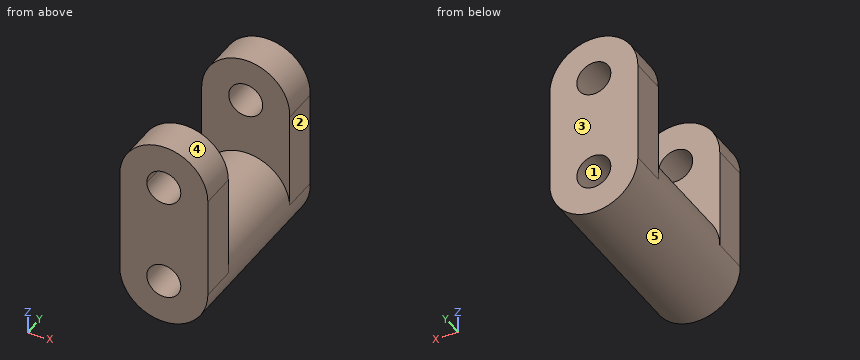
from build123d import *

# Parameters (mm, degrees)
F0_R     = 29.837596
F1_DEPTH = 127
F3_DEPTH = 25.4
F5_DEPTH = 25.4
F6_R     = 11.514098
F7_DEPTH = 249.174


with BuildPart() as f1:
    # F0 (on Front) → F1 (new body)
    with BuildSketch(Plane.XZ):
        with Locations((0, -34.119722)):
            Circle(F0_R)
    extrude(amount=F1_DEPTH)

    # F2 (on face) → F3 (join)
    with BuildSketch(Plane.XZ.offset(127)):
        with BuildLine():
            Line((-11.514098, -34.119722), (0, -34.119722))
            Line((0, -34.119722), (11.514098, -34.119722))
            ThreePointArc((11.514098, -34.119722), (0, -22.605623), (-11.514098, -34.119722))
        make_face()
        with BuildLine():
            Line((-29.837596, -34.119722), (-11.514098, -34.119722))
            ThreePointArc((-11.514098, -34.119722), (0, -22.605623), (11.514098, -34.119722))
            Line((11.514098, -34.119722), (29.837596, -34.119722))
            ThreePointArc((29.837596, -34.119722), (0, -4.282125), (-29.837596, -34.119722))
        make_face()
        with BuildLine():
            Line((-29.837596, 34.119722), (-29.837596, -34.119722))
            ThreePointArc((-29.837596, -34.119722), (0, -4.282125), (29.837596, -34.119722))
            Line((29.837596, -34.119722), (29.837596, 34.119722))
            ThreePointArc((29.837596, 34.119722), (0, 63.957318), (-29.837596, 34.119722))
        make_face()
        with BuildLine():
            ThreePointArc((11.514098, 34.119722), (0, 22.605623), (-11.514098, 34.119722))
            ThreePointArc((-11.514098, 34.119722), (0, 45.63382), (11.514098, 34.119722))
        make_face(mode=Mode.SUBTRACT)
    extrude(amount=-F3_DEPTH)

    # F4 (on face) → F5 (join)
    with BuildSketch(Plane(origin=(0, 0, 0), x_dir=(-1, 0, 0), z_dir=(0, 1, 0))):
        with BuildLine():
            Line((-29.798884, -34.119722), (0, -34.119722))
            Line((0, -34.119722), (29.416961, -34.119722))
            Line((29.416961, -34.119722), (29.837596, -34.119722))
            Line((29.837596, -34.119722), (29.837596, -29.127271))
            Line((29.837596, -29.127271), (29.837596, 33.523746))
            ThreePointArc((29.837596, 33.523746), (-0.759963, 63.351663), (-29.798884, 32.004312))
            Line((-29.798884, 32.004312), (-29.798884, -34.119722))
        make_face()
    extrude(amount=-F5_DEPTH)

    # F6 (on face) → F7 (cut)
    with BuildSketch(Plane.XZ.offset(127)):
        with Locations((0, 34.119722)):
            Circle(F6_R)
        with Locations((0, -34.119722)):
            Circle(F6_R)
    extrude(amount=-F7_DEPTH, mode=Mode.SUBTRACT)


solid = f1.part
Check sheet for the modelled part. Datum: model origin and axes. Units: mm. Face numbers are marked on the shaded views. A direction names the side the tool comes from. Give positions to 0.01 mm unless a question says otherwise; leave off trailing zeros. Write each loop counter-clockwise with the first axis right and the second up, starting at its lowest first coordinate (ties: lowest second). Pieces come first, ordered by that corner, then holes. Notation, with made-up numbers: (84.25, 9) -> (114.25, 9) arc R16 ccw to (114.25, 18) -> close; hole circle Ø3 at (67.5, 17). An arc over 180 degrees is marked (long way). Use one line per item in the form item = value. Start each with the question number.
1. Go/stop test with flat-tipped pins: P1, Ø10, axis at x = 11.5, y = -104, coming from the +Z side; P2, Ø3, axis at x = 20.5, y = -69, coming from the -Z side; P3, Ø20.5, axis at x = 0, z = 34.12, coming from the +Y side; P4, Ø6, axis at x = -4.5, y = -21.5, coming from the +Z side. Record where each tip stops, or that it passes through.
2. Section check A-A (x = 0). Record the cut outline in (y, z), and give its area (3 significant figures).
3. Section check B-B (z = 14.5). Record the cut outline in (x, y).
4. Section check D-D (z = 55). Record the cut outline in (x, y).
5. Section check C-C (y = -20.5). Record the cut outline in (x, z).
6. Thickness scan on line 1 along Z through (x, y) = (0, -74); line 2 along Y through (x, z) = (-13.5, 57.5); line 3 along Z through (x, y) = (0, -18.5). Record the ranges inside material, lowest first. Write a range as from..to.
7. Mould release check, pull along X, two halves, no side actions. Record for the marked faces 1, 2 and 3: pulls with the +X half, pulls with the -X half, needs draft (parallel to the pull), parting line crosses it, or undercut.
8. Access from +Z, -Z, +X, -X, +Y, -Y to the whole of each face (thin tool, end or side, straight path). Record for the marked faces 4 and 5.
Conclusion:
q1.P1 = 63.24
q1.P2 = -57.13
q1.P3 = through
q1.P4 = 63.32
q2.outline = (-127, -63.96) -> (0, -63.96) -> (0, -45.63) -> (-127, -45.63) -> close; (-127, -22.61) -> (0, -22.61) -> (0, 22.61) -> (-25.4, 22.61) -> (-25.4, -4.28) -> (-101.6, -4.28) -> (-101.6, 22.61) -> (-127, 22.61) -> close; (-127, 45.63) -> (-101.6, 45.63) -> (-101.6, 63.96) -> (-127, 63.96) -> close; (-25.4, 45.63) -> (0, 45.63) -> (0, 63.36) -> (-25.4, 63.36) -> close
q2.area = 6,940 mm²
q3.outline = (-29.84, -127) -> (29.84, -127) -> (29.84, -101.6) -> (-29.84, -101.6) -> close; (-29.84, -25.4) -> (29.8, -25.4) -> (29.8, 0) -> (-29.84, 0) -> close
q4.outline = (-21.31, -127) -> (21.31, -127) -> (21.31, -101.6) -> (-21.31, -101.6) -> close; (-20.71, -25.4) -> (20.71, -25.4) -> (20.71, 0) -> (-20.71, 0) -> close
q5.outline = (-29.84, -34.12) arc R29.84 ccw (long way) to (29.8, -32.6) -> (29.8, 32) arc R29.84 ccw (long way) to (-29.84, 33.52) -> close; hole circle Ø23.03 at (0, -34.12); hole circle Ø23.03 at (0, 34.12)
q6.line_1 = -63.96..-45.63, -22.61..-4.28
q6.line_2 = -127..-101.6, -25.4..0
q6.line_3 = -63.96..-45.63, -22.61..22.61, 45.63..63.36
q7.face_1 = undercut
q7.face_2 = pulls with the +X half
q7.face_3 = needs draft
q8.face_4 = +Z, +Y, -Y
q8.face_5 = none
